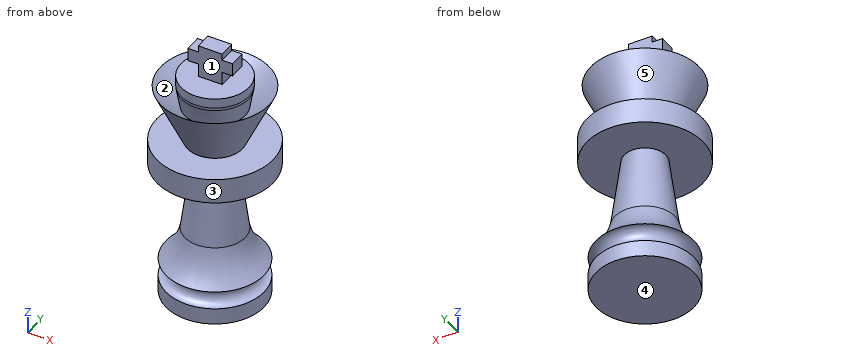
```python
from build123d import *

# Parameters (mm, degrees)
F1_FACE_R = 15
F2_DEPTH  = 5
F3_DEPTH  = 2.5
F4_DEPTH  = 2.5
F5_R      = 5


with BuildPart() as f1:
    # F0 (on Front) → F1 (revolve)
    with BuildSketch(Plane.XZ):
        with BuildLine():
            Line((0, 65.57779), (0, 0))
            Line((0, 0), (15, 0))
            ThreePointArc((15, 0), (12.238, 2.762), (15, 5.524))
            ThreePointArc((15, 5.524), (11.27401, 10.147038), (9.206386, 15.713044))
            Line((9.206386, 15.713044), (6.373653, 36.958547))
            Line((6.373653, 36.958547), (17.772784, 36.958547))
            Line((17.772784, 36.958547), (17.772784, 44.600636))
            Line((17.772784, 44.600636), (8.38892, 44.600636))
            Line((8.38892, 44.600636), (16.571492, 62.178511))
            Line((16.571492, 62.178511), (9.241848, 55.88216))
            Line((9.241848, 55.88216), (10.373653, 62.178511))
            Line((10.373653, 62.178511), (10.373653, 65.57779))
            Line((10.373653, 65.57779), (3.642126, 65.57779))
            Line((3.642126, 65.57779), (0, 65.57779))
        make_face()
    revolve(axis=Axis((0, 0, 32.788895), (0, 0, 1)))

    # F1_face (on face) → F2 (join)
    with BuildSketch(Plane(origin=(0, 0, 0), x_dir=(1, 0, 0), z_dir=(0, 0, -1))):
        Circle(F1_FACE_R)
    extrude(amount=F2_DEPTH)

    # F0 (on Front) → F3 (join)
    with BuildSketch(Plane.XZ):
        Polygon((-3.642126, 65.57779), (0, 65.57779), (3.642126, 65.57779), (3.642126, 69.57779), (6.778388, 69.57779), (6.778388, 73.57779), (3.642126, 73.57779), (3.642126, 75.57779), (0, 75.57779), (-3.642126, 75.57779), (-3.642126, 73.57779), (-6.778388, 73.57779), (-6.778388, 69.57779), (-3.642126, 69.57779), align=None)
    extrude(amount=F3_DEPTH)

    # F0 (on Front) → F4 (join)
    with BuildSketch(Plane.XZ):
        Polygon((-3.642126, 65.57779), (0, 65.57779), (3.642126, 65.57779), (3.642126, 69.57779), (6.778388, 69.57779), (6.778388, 73.57779), (3.642126, 73.57779), (3.642126, 75.57779), (0, 75.57779), (-3.642126, 75.57779), (-3.642126, 73.57779), (-6.778388, 73.57779), (-6.778388, 69.57779), (-3.642126, 69.57779), align=None)
    extrude(amount=-F4_DEPTH)

    # F5
    f5_edges = [f1.edges().sort_by_distance(p)[0] for p in [
        (-10.373653, 0, 62.178511),
    ]]
    fillet(f5_edges, radius=F5_R)


solid = f1.part
```
CAD build for the part. Positions are in the model's coordinates, mm. Face numbers are marked on the shaded views. A direction names the side the tool comes from. Give positions to 0.01 mm unless a question says otherwise; leave off trailing zeros. Order: outer loops, then holes, each group sorted by start corner. A loop starts at its lowest first (then second) coordinate and runs counter-clockwise, first axis right, second up. Notation, with made-up numbers: M 24,56.5 L 76,56.5 A19 cw 76,71.5 Z; hole C -24.5,20.25 d9. An arc over 180 degrees is marked long. Put each result on its own line as item: value. Start each with the question number.
(1) Flat gauge pins, fed straight in: pin 1 Ø11 at (x, z) = (-3, 73) entering from -Y; pin 2 Ø2.5 at (x, y) = (-6, 0.5) entering from +Z; pin 3 Ø1.2 at (y, z) = (0, 68) entering from +X. Where does each tip first touch, or does it go through?
(2) Drill centre lines: line 1 along Z through (x, y) = (-1, 11.5); line 2 along Z through (x, y) = (-2, -11.5); line 3 along Z through (x, y) = (-2, -13). Where is each one in solid material? Low to high.
(3) Saw through at C-C, the plane x = 11.5. Give the number of separate pieces and of enclosed holes in the cut face, then the cut area to 3 significant figures.
(4) Saw through at A-A, the plane z = 57.5. Write the cut outline in (x, y), then the cut area to 3 significant figures.
(5) Saw through at B-B, the plane z = 67.5. Write the cut outline in (x, y).
(6) Mould opens along X. For the marked faces 1, 2 and 3 say: +X half, -X half, draft (parallel to the pull), parting line (faces both ways), or undercut.
(7) Which spindle directions (+Z, -Z, +X, -X, +Y, -Y) get a long thin tool onto all of the face, cutting with end or side? Do the marked faces 4 and 5. Say none if no direction does.
Check result:
1. pin 1: stops at y = -2.5
1. pin 2: stops at z = 73.58
1. pin 3: stops at x = 3.64
2. line 1: z = -5 to 9.69, 36.96 to 44.6, 51.38 to 57.86
2. line 2: z = -5 to 9.48, 36.96 to 44.6, 51.65 to 57.97
2. line 3: z = -5 to 0.71, 4.82 to 7.44, 36.96 to 44.6, 54.83 to 59.24
3. separate pieces: 3
3. enclosed holes: 0
3. area: 515 mm2
4. outline: C 0,0 d28.79; C 0,0 d19.07; hole C 0,0 d22.25
4. area: 548 mm2
5. outline: M -3.64,-2.5 L 3.64,-2.5 L 3.64,2.5 L -3.64,2.5 Z
6. face 1: draft
6. face 2: undercut
6. face 3: parting line
7. face 4: -Z, +X, -X, +Y, -Y
7. face 5: none
